Part model, mm, in its own coordinate system. Face numbers are marked on the shaded views. A direction names the side the tool comes from. Give positions to 0.01 mm unless a question says otherwise; leave off trailing zeros. Order: outer loops, then holes, each group sorted by start corner. A loop starts at its lowest first (then second) coordinate and runs counter-clockwise, first axis right, second up. Notation, with made-up numbers: (28.5, 58.25) -> (54.5, 58.25) arc R14 cw to (54.5, 65.25) -> close; hole circle Ø11 at (-2.5, 38). An arc over 180 degrees is marked (long way). Write item = value, one per line. Start each with the question number.
Item 1: Band-saw the part on A-A on z = 2. Write the cut outline in (x, y).
Item 2: Band-saw the part on B-B on x = 3.75. Write the cut outline in (y, z), plus the area to 3 significant figures.
Item 3: Flat gauge pins, fed straight in: P1, Ø8, axis at x = 0, z = 0, coming from the -Y side; P2, Ø2, axis at y = -15.5, z = 5.5, coming from the -X side; P3, Ø6.5, axis at x = -8.5, y = -10, coming from the -Z side; P4, Ø4, axis at y = -5.5, z = 8.5, coming from the -X side. Where does each tip first touch, or does it go through?
Item 4: Pull direction Z, two halves, no side cores. Call the marked faces 3, 4 and 5: +Z half, -Z half, draft (parallel to the pull), parting line (faces both ways), or undercut.
Item 5: Tool access for the marked faces 1 and 2: list every direction of +Z, -Z, +X, -X, +Y, -Y with a clear straight run to the whole face (end or side of a thin tool).
Item 6: Band-saw the part on D-D on z = -9.5. Write the cut outline in (x, y).
Item 7: Band-saw the part on C-C on y = -23.5. Write the cut outline in (x, z), plus the area to 3 significant figures.
Item 8: Drill centre lines: line 1 along Y through (x, z) = (-7.25, -3.75); line 2 along Z through (x, y) = (0, -18.5); line 3 along X through (y, z) = (-6.5, 4.5). Where is each one in solid material? Low to high.
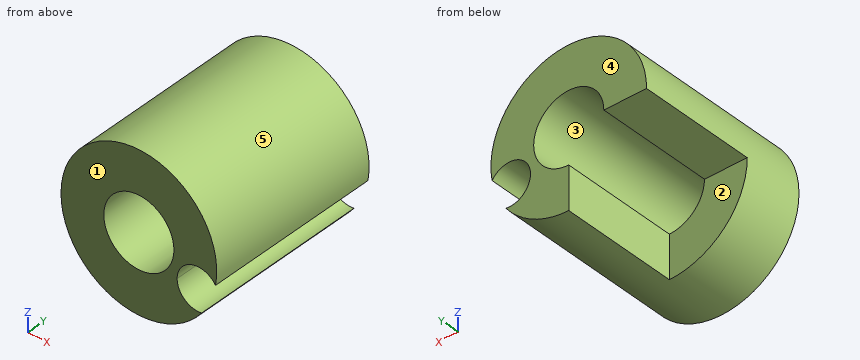
```python
from build123d import *

# Parameters (mm, degrees)
F0_R     = 11.1
F0_R_2   = 5
F1_DEPTH = 25.4
F2_W     = 16.7754087597
F2_H     = 27.2372085601
F3_DEPTH = 76.2
F5_DEPTH = 25.401


with BuildPart() as f1:
    # F0 (on Front) → F1 (new body)
    with BuildSketch(Plane.XZ):
        Circle(F0_R)
        Circle(F0_R_2, mode=Mode.SUBTRACT)
    extrude(amount=F1_DEPTH)

    # F2 (on Right) → F3 (cut)
    with BuildSketch(Plane.YZ):
        with Locations((-8.3877043799, -13.6186042801)):
            Rectangle(F2_W, F2_H)
    extrude(amount=-F3_DEPTH, mode=Mode.SUBTRACT)

    # F4 (on face) → F5 (cut, through all)
    with BuildSketch(Plane(origin=(0, 0, 0), x_dir=(-1, 0, 0), z_dir=(0, 1, 0))):
        with BuildLine():
            ThreePointArc((-8.9445990977, -6.572986154), (-6.5138225835, -5.901619973), (-5.4539214149, -3.6133856047))
            ThreePointArc((-5.4539214149, -3.6133856047), (-7.5692818154, -0.7467826013), (-10.9321966009, -1.9227785828))
            ThreePointArc((-10.9321966009, -1.9227785828), (-10.2067555778, -4.3625841625), (-8.9445990977, -6.572986154))
        make_face()
    extrude(amount=-F5_DEPTH, mode=Mode.SUBTRACT)


solid = f1.part
```
Values found:
q1.outline = (-10.92, -25.4) -> (-4.58, -25.4) -> (-4.58, 0) -> (-10.92, 0) -> close; (4.58, -25.4) -> (10.92, -25.4) -> (10.92, 0) -> (4.58, 0) -> close
q2.outline = (-25.4, -10.45) -> (0, -10.45) -> (0, -3.31) -> (-25.4, -3.31) -> close; (-25.4, 3.31) -> (0, 3.31) -> (0, 10.45) -> (-25.4, 10.45) -> close
q2.area = 363 mm^2
q3.P1 = through
q3.P2 = -10.15
q3.P3 = 0
q3.P4 = -9
q4.face_3 = undercut
q4.face_4 = draft
q4.face_5 = parting line
q5.face_1 = +Z, -Z, +X, -X, -Y
q5.face_2 = -Z, -X, +Y
q6.outline = (-5.74, -25.4) -> (5.74, -25.4) -> (5.74, 0) -> (0, 0) -> (0, -16.78) -> (-5.74, -16.78) -> close
q7.outline = (8.94, -6.57) arc R3 cw (long way) to (10.93, -1.92) arc R11.1 ccw (long way) to start; hole circle Ø10 at (0, 0)
q7.area = 284 mm^2
q8.line_1 = -25.4 to -16.78
q8.line_2 = -11.1 to -5, 5 to 11.1
q8.line_3 = -10.15 to -2.18, 2.18 to 10.15
